```python
from build123d import *

# Parameters (mm, degrees)
F0_R     = 6.0248478502
F0_R_2   = 6.5557456881
F1_DEPTH = 6.35
F0_W     = 4.6359449625
F0_H     = 22.1776319668
F2_DEPTH = 25.4


with BuildPart() as f1:
    # F0 (on Top) → F1 (new body)
    with BuildSketch(Plane.XY):
        with BuildLine():
            ThreePointArc((-12.6521838829, 25.6658587605), (-24.7018816881, 37.7155565657), (-36.7515794933, 25.6658587605))
            Line((-36.7515794933, 25.6658587605), (-36.7515794933, -20.6049848348))
            ThreePointArc((-36.7515794933, -20.6049848348), (-24.7018816881, -32.65468264), (-12.6521838829, -20.6049848348))
            Line((-12.6521838829, -20.6049848348), (-12.6521838829, 25.6658587605))
        make_face()
        with Locations((-24.7018816881, -20.6049848348)):
            Circle(F0_R, mode=Mode.SUBTRACT)
        Polygon((-25.1393578947, 14.3663082272), (-20.5034129322, 14.3663082272), (-20.5034129322, -7.8113237396), (-25.1393578947, -7.8113237396), (-29.7753028572, -7.8113237396), (-29.7753028572, 14.3663082272), align=None, mode=Mode.SUBTRACT)
        with Locations((-24.7018816881, 25.6658587605)):
            Circle(F0_R_2, mode=Mode.SUBTRACT)
    extrude(amount=F1_DEPTH)

    # F0 (on Top) → F2 (join)
    with BuildSketch(Plane.XY):
        with Locations((-22.8213854134, 3.2774922438)):
            Rectangle(F0_W, F0_H)
        with Locations((-27.4573303759, 3.2774922438)):
            Rectangle(F0_W, F0_H)
    extrude(amount=F2_DEPTH)


solid = f1.part
```
Check sheet for the modelled part. Datum: model origin and axes. Units: mm. A direction names the side the tool comes from. Give positions to 0.01 mm unless a question says otherwise; leave off trailing zeros. Order: outer loops, then holes, each group sorted by start corner. A loop starts at its lowest first (then second) coordinate and runs counter-clockwise, first axis right, second up. Notation, with made-up numbers: (13, -5.5) -> (26, -5.5) arc R13 cw to (26, 19.5) -> close; hole circle Ø5 at (76.5, -33.5). An arc over 180 degrees is marked (long way). Return JSON: item names as keys, results as strings.
1. Cross-section at B-B, the plane z = 2.75. Record the cut outline in (x, y).
From the geometry:
{"outline": "(-36.75, -20.6) arc R12.05 ccw to (-12.65, -20.6) -> (-12.65, 25.67) arc R12.05 ccw to (-36.75, 25.67) -> close; hole circle Ø13.11 at (-24.7, 25.67); hole circle Ø12.05 at (-24.7, -20.6)"}
2. Mould release check, pull along X, two halves, no side actions. Record for faces 6 (the cylindrical face through (-24.97, -32.65, 3.13)), 7 (the flat face through (-36.752, 3, 3)), 8 (the cylindrical face through (-18.955, -18.795, 3.131)), 9 (the cylindrical face through (-18.45, 27.64, 3.13)): +X half, -X half, draft (parallel to the pull), parting line (faces both ways), or undercut.
From the geometry:
{"face 6": "parting line", "face 7": "-X half", "face 8": "undercut", "face 9": "undercut"}
3. Material ranges on probe 1 along Z at (x, y) = (-14, -7); probe 2 along Y at (x, z) = (-27.25, 21.25); probe 3 along X at (y, z) = (-5, 10.25), recorded low to high. Write a range as [from, to].
From the geometry:
{"probe 1": "[0, 6.35]", "probe 2": "[-7.81, 14.37]", "probe 3": "[-29.78, -20.5]"}
4. Cross-section at C-C, the plane y = -24.5. Record the cut outline in (x, z).
From the geometry:
{"outline": "(-36.1, 0) -> (-29.3, 0) -> (-29.3, 6.35) -> (-36.1, 6.35) -> close; (-20.11, 0) -> (-13.3, 0) -> (-13.3, 6.35) -> (-20.11, 6.35) -> close"}
5. Set-up check for faces 1 (the flat face through (-29.775, 3, 16)), 2 (the flat face through (-25, 14.366, 16)), 3 (the flat face through (-25, -7.811, 16)), 4 (the flat face through (-25, 3, 25.4)), 5 (the flat face through (-20.503, 3, 16)): record each of +Z, -Z, +X, -X, +Y, -Y from which the full face is reachable in a straight line by a thin tool's end or side.
From the geometry:
{"face 1": "+Z, -X, +Y, -Y", "face 2": "+Z, +X, -X, +Y", "face 3": "+Z, +X, -X, -Y", "face 4": "+Z, +X, -X, +Y, -Y", "face 5": "+Z, +X, +Y, -Y"}
6. Cross-section at A-A, the plane x = -19.5. Record the cut outline in (y, z), plus the area to 3 significant figures.
From the geometry:
{"outline": "(-31.47, 0) -> (-23.64, 0) -> (-23.64, 6.35) -> (-31.47, 6.35) -> close; (-17.57, 0) -> (21.68, 0) -> (21.68, 6.35) -> (-17.57, 6.35) -> close; (29.66, 0) -> (36.53, 0) -> (36.53, 6.35) -> (29.66, 6.35) -> close", "area": "343 mm^2"}
7. Cross-section at D-D, the plane y = 7. Record the cut outline in (x, z), plus the area to 3 significant figures.
From the geometry:
{"outline": "(-36.75, 0) -> (-12.65, 0) -> (-12.65, 6.35) -> (-20.5, 6.35) -> (-20.5, 25.4) -> (-29.78, 25.4) -> (-29.78, 6.35) -> (-36.75, 6.35) -> close", "area": "330 mm^2"}
8. Go/stop test with flat-tipped pins: P1, Ø3, axis at x = -23, z = 13.5, coming from the +Y side; P2, Ø5, axis at x = -34, y = 10.5, coming from the +Z side; P3, Ø6, axis at x = -32.5, z = 17.5, coming from the -Y side. Record where each tip stops, or that it passes through.
From the geometry:
{"P1": "y = 14.37", "P2": "z = 6.35", "P3": "y = -7.81"}
